```python
from build123d import *

# Parameters (mm, degrees)
SKETCH2_R          = 8
CUT_EXTRUDE1_DEPTH = 3
SKETCH3_R          = 2.5
CUT_EXTRUDE2_DEPTH = 0.01


with BuildPart() as part:
    # Sketch1 → Revolve1 (revolve)
    with BuildSketch(Plane(origin=(0, 0, 0), x_dir=(0, 0, -1), z_dir=(1, 0, 0))):
        Polygon((0, 32), (0, -32), (-3.25, -32), (-10.9, -26.023164957), (-10.9, -24.5), (-12.4, -24.5), (-12.9, -24), (-12.9, -19.7), (-14, -19.7), (-14, -16.7), (-16.5, -14.2), (-16.5, 21.5), (-15.683726929, 21.5), (-15.683726929, 21.75), (-14.25, 26.75), (-14, 26.75), (-14, 27), (-11.9, 27), (-11.9, 28), (-12.5, 28.6), (-12.5, 30.4), (-11.9, 31), (-11.9, 32), align=None)
    revolve(axis=Axis((0, 40, 0), (0, -1, 0)))

    # Sketch2 → Cut-Extrude1 (cut)
    with BuildSketch(Plane(origin=(0, 32, 0), x_dir=(1, 0, 0), z_dir=(0, 1, 0))):
        with Locations(Location((0, 0, 0), (0, 0, 270))):
            Circle(SKETCH2_R)
    extrude(amount=-CUT_EXTRUDE1_DEPTH, mode=Mode.SUBTRACT)

    # Sketch3 → Cut-Extrude2 (cut)
    with BuildSketch(Plane(origin=(0, -32, 0), x_dir=(-1, 0, 0), z_dir=(0, -1, 0))):
        with Locations(Location((0, 0, 0), (0, 0, 90))):
            Circle(SKETCH3_R)
    extrude(amount=-CUT_EXTRUDE2_DEPTH, mode=Mode.SUBTRACT)


solid = part.part
```
Part model, mm, in its own coordinate system. A direction names the side the tool comes from. Round coordinates to 2 decimals unless told otherwise and drop trailing zeros. Order: outer loops, then holes, each group sorted by start corner. A loop starts at its lowest first (then second) coordinate and runs counter-clockwise, first axis right, second up. Notation, with made-up numbers: M 33,75 L 86,75 A23 cw 86,106 Z; hole C 68,33.25 d3. An arc over 180 degrees is marked long. Answer in a Markdown table with one row per item. Add a question column.
Q1. Cut at B-B on y = 17.5. Give the cut face in (x, z).
Q2. 3-axis set-ups, long thin cutter, end or side, ignore diameter. For faces 1 (the face through (10.3, 27, -6.3)), 2 (the face through (12.593, -21.82, -2.796)), 3 (the face through (6, 21.5, 15)): which of +Z, -Z, +X, -X, +Y, -Y reach the whole face in a straight line?
Q3. Mould opens along Z. For faces 4 (the face through (-7.81, 30.52, -1.73)), 5 (the face through (4.1, -19.7, -12.4)), 6 (the face through (-8.043, 27.507, -8.771)) say: +Z half, -Z half, draft (parallel to the pull), parting line (faces both ways), or undercut.
Q4. Cut at A-A on y = -20.5. Give the cut face in (x, z).
Q5. Pin check, flat tips, straight feed: pin 1 (8 mm diameter, centred on x = 13, y = -11, fed in from -Z); pin 2 (2 mm diameter, centred on x = 6.5, y = -22.5, fed in from +Z); pin 3 (4 mm diameter, centred on x = 8.5, z = -7.5, fed in from -Y). Stop position of each tip, or through.
Q6. Wall check: L1, parallel to X at y = 31, z = 0; L2, parallel to Y at x = 10.5, z = 5; L3, parallel to Y at x = 3, z = 12. Give the ranges that are in metal, low to high. Write a range as from..to.
Established:
| question | item | result |
|---|---|---|
| 1 | outline | C 0,0 d33 |
| 2 | face 1 | none |
| 2 | face 2 | -Y |
| 2 | face 3 | +Y |
| 3 | face 4 | undercut |
| 3 | face 5 | draft |
| 3 | face 6 | parting line |
| 4 | outline | C 0,0 d25.8 |
| 5 | pin 1 | stops at z = -13.83 |
| 5 | pin 2 | stops at z = 11.67 |
| 5 | pin 3 | stops at y = -27.25 |
| 6 | L1 | x = -11.9..-8, 8..11.9 |
| 6 | L2 | y = -24.5..32 |
| 6 | L3 | y = -24.5..27, 28.47..30.53 |
